Could you check a few things on this model? Use its own coordinates, in mm. A direction names the side the tool comes from. Coordinates: 2 decimals unless noted, no trailing zeros. Loops run counter-clockwise (first coordinate to the right, second up) from the corner with the lowest first, then second, coordinate; pieces in that order, holes last. Notation, with made-up numbers: (67, -36) -> (72, -36) arc R26 ccw to (72, 3) -> close; hole circle Ø5 at (-35.5, 69). An arc over 180 degrees is marked (long way). One line per question, with ' | ' between items.
```python
from build123d import *

# Parameters (mm, degrees)
EXTRUDE_2_DEPTH          = 2.5
EXTRUDE_3_DEPTH          = 3
CUT_EXTRUDE_1_DEPTH      = 77.94617208
CUT_EXTRUDE_1_DEPTH_BACK = 77.94617208
SKETCH_5_R               = 2
FILLET_1_R               = 10
FILLET_2_R               = 8
FILLET_3_R               = 8


with BuildPart() as part:
    # 草图1 → 凸台-拉伸2 (new body)
    with BuildSketch(Plane.XY.offset(5.5)):
        with BuildLine():
            Line((-41.12, -13.858374143), (41.12, -13.858374143))
            Line((41.12, -13.858374143), (61.27, -2.231637876))
            ThreePointArc((61.27, -2.231637876), (73.122690209, 2.892045504), (62.764706552, -4.818374143))
            Line((62.764706552, -4.818374143), (41.92, -16.858374143))
            Line((41.92, -16.858374143), (-41.92, -16.858374143))
            Line((-41.92, -16.858374143), (-62.77, -4.818374143))
            ThreePointArc((-62.77, -4.818374143), (-73.132598603, 2.884045772), (-61.27, -2.213941747))
            Line((-61.27, -2.213941747), (-41.12, -13.858374143))
        make_face()
    extrude(amount=EXTRUDE_2_DEPTH)

    # 草图4 → 凸台-拉伸3 (add)
    with BuildSketch(Plane.XY.offset(8)):
        with BuildLine():
            Line((-61.14, 0.981789849), (-40.05, -10.358374143))
            Line((-40.05, -10.358374143), (40.31, -10.358374143))
            Line((40.31, -10.358374143), (61.134706552, 0.981789849))
            ThreePointArc((61.134706552, 0.981789849), (72.181493512, 4.143779301), (68.582245444, -6.768374143))
            Line((68.582245444, -6.768374143), (42.99, -20.358374143))
            Line((42.99, -20.358374143), (-42.73, -20.358374143))
            Line((-42.73, -20.358374143), (-66.412461108, -6.768374143))
            ThreePointArc((-66.412461108, -6.768374143), (-72.874264542, 3.296129187), (-61.14, 0.981789849))
        make_face()
    extrude(amount=EXTRUDE_3_DEPTH)

    # 草图5 → 切除-拉伸1 (cut, two sides: drawn at the far end of the back side and taken through both)
    with BuildSketch(Plane.XY.offset(11).offset(-CUT_EXTRUDE_1_DEPTH_BACK)):
        with Locations((67.494706552, -0.36)):
            Circle(SKETCH_5_R)
        with Locations((-67.5, -0.36)):
            Circle(SKETCH_5_R)
    extrude(amount=CUT_EXTRUDE_1_DEPTH + CUT_EXTRUDE_1_DEPTH_BACK, mode=Mode.SUBTRACT)

    # 圆角1
    fillet_1_edges = [part.edges().sort_by_distance(p)[0] for p in [
        (41.92, -16.858374143, 6.75),
        (-41.92, -16.858374143, 6.75),
        (-42.73, -20.358374143, 9.5),
        (42.99, -20.358374143, 9.5),
    ]]
    fillet(fillet_1_edges, radius=FILLET_1_R)

    # 圆角2
    fillet_2_edges = [part.edges().sort_by_distance(p)[0] for p in [
        (61.27, -2.231637876, 6.75),
        (62.764706552, -4.818374143, 6.75),
        (-62.77, -4.818374143, 6.75),
        (-61.27, -2.213941747, 6.75),
    ]]
    fillet(fillet_2_edges, radius=FILLET_2_R)

    # 圆角3
    fillet_3_edges = [part.edges().sort_by_distance(p)[0] for p in [
        (-41.12, -13.858374143, 6.75),
        (41.12, -13.858374143, 6.75),
        (40.31, -10.358374143, 9.5),
        (-40.05, -10.358374143, 9.5),
    ]]
    fillet(fillet_3_edges, radius=FILLET_3_R)


solid = part.part
```
Q1. For faces 1 (the face through (-51.398, -11.385, 6.732)), 2 (the face through (1, -18, 8)), 3 (the face through (0, -10.358, 9)), 4 (the face through (0, -11, 8)), which set-ups out of +Z, -Z, +X, -X, +Y, -Y let a thin tool reach every point of the face, with its end or its side?
Values follow:
face 1: -Z, -X, -Y | face 2: -Z, -Y | face 3: +Z, -Z, +Y | face 4: -Z, +Y
Q2. Imagine slicing it at A-A on z = 6.85. Write out the boundary of the cut face in (x, y).
Values follow:
outline: (-65.37, -6.5) arc R8 cw to (-58.76, -7.14) -> (-44.24, -15.52) arc R10 ccw to (-39.24, -16.86) -> (39.24, -16.86) arc R10 ccw to (44.24, -15.52) -> (58.75, -7.14) arc R8 cw to (65.37, -6.5) arc R6.5 ccw (long way) to (61.11, 0.87) arc R8 cw to (57.25, -4.55) -> (42.98, -12.79) arc R8 cw to (38.98, -13.86) -> (-38.97, -13.86) arc R8 cw to (-42.98, -12.78) -> (-57.27, -4.53) arc R8 cw to (-61.12, 0.88) arc R6.5 ccw (long way) to start; hole circle Ø4 at (-67.5, -0.36); hole circle Ø4 at (67.49, -0.36)
Q3. Imagine slicing it at C-C on x = -10. Write out the boundary of the cut face in (y, z).
Values follow:
outline: (-20.36, 8) -> (-16.86, 8) -> (-16.86, 5.5) -> (-13.86, 5.5) -> (-13.86, 8) -> (-10.36, 8) -> (-10.36, 11) -> (-20.36, 11) -> close
Q4. Imagine slicing it at B-B on y = -0.36. Write out the boundary of the cut face in (x, z), plus the area to 3 significant figures.
Values follow:
outline: (-74, 5.5) -> (-69.5, 5.5) -> (-69.5, 11) -> (-74, 11) -> close; (-65.5, 5.5) -> (-60.77, 5.5) -> (-60.77, 8) -> (-58.64, 8) -> (-58.64, 11) -> (-65.5, 11) -> close; (58.67, 8) -> (60.77, 8) -> (60.77, 5.5) -> (65.49, 5.5) -> (65.49, 11) -> (58.67, 11) -> close; (69.49, 5.5) -> (73.99, 5.5) -> (73.99, 11) -> (69.49, 11) -> close | area: 114 mm2
Q5. Please list where these lines run through material, in increasing order: L1, parallel to Y at x = -67.5, z = 9.1; L2, parallel to X at y = 1, z = 7.5; L3, parallel to X at y = -0.36, z = 7.4. Write a range as [from, to].
Values follow:
L1: y = [-6.86, -2.36], [1.64, 6.14] | L2: x = [-73.86, -68.97], [-66.03, -61.14], [61.14, 66.03], [68.96, 73.85] | L3: x = [-74, -69.5], [-65.5, -60.77], [60.77, 65.49], [69.49, 73.99]
Q6. Imagine slicing it at D-D on x = -64. Write out the boundary of the cut face in (y, z), plus the area to 3 significant figures.
Values follow:
outline: (-8.15, 8) -> (-6.16, 8) -> (-6.16, 5.5) -> (5.12, 5.5) -> (5.12, 11) -> (-8.15, 11) -> close | area: 68.0 mm2
Q7. For pin 1 (3 mm diameter, centred on y = -7, z = 9, fed in from +X); pin 2 (1.5 mm diameter, centred on y = -2, z = 6.5, fed in from +X); pin 3 (0.8 mm diameter, centred on x = 3.5, z = 6.5, fed in from -Y), each with a flat end and sliding along its axis, tell me the tip position at first contact or that it passes through.
Values follow:
pin 1: stops at x = 71.47 | pin 2: stops at x = 73.93 | pin 3: stops at y = -16.86
Q8. We'd pull the mould along X, two halves only. Please class faces 5 (the face through (1, -16.858, 7)), 6 (the face through (-51.617, -4.139, 9.479)), 7 (the face through (57.05, -12.89, 9.48)): released by +X, released by -X, zero draft, split by the parting line, or undercut.
Values follow:
face 5: zero draft | face 6: undercut | face 7: released by +X
